Autodesk Inventor part; units mm, degrees
ref_plane "YZ Plane" through (0, 0, 0) normal (1, 0, 0) x (0, 1, 0)
ref_plane "XZ Plane" through (0, 0, 0) normal (0, 1, 0) x (-1, 0, 0)
ref_plane "XY Plane" through (0, 0, 0) normal (0, 0, 1) x (1, 0, 0)
sketch "Sketch1" plane through (0, 0, 0) normal (0, 0, 1) x (1, 0, 0)
  line L0 (0, 0) -> (30, 0)
  line L1 (30, 0) -> (30, 27)
  line L2 (30, 27) -> (0, 27)
  line L3 (0, 27) -> (0, 0)
  dimension "d0" = 30
  dimension "d1" = 27
extrude "Extrusion1" add sketch "Sketch1" along normal blind 3
sketch "Sketch2" plane through (0, 27, 0) normal (0, 1, 0) x (1, 0, 0)
  line L0 (0, 0) -> (0, -3)
  line L1 (0, 0) -> (30, 0)
  line L2 (0, -3) -> (10, -3)
  line L3 (10, -3) -> (10, 0)
  line L4 (10, 0) -> (0, 0)
  line L5 (0, 0) -> (0, -3)
  dimension "d4" = 10
extrude "Extrusion2" add sketch "Sketch2" along normal blind 2
sketch "Sketch3" plane through (0, 29, 0) normal (0, 1, 0) x (1, 0, 0)
  line L0 (0, 0) -> (0, -3)
  line L1 (0, -3) -> (32, -3)
  line L2 (32, -3) -> (32, 0)
  line L3 (32, 0) -> (0, 0)
  line L4 (0, 0) -> (0, -3)
  point P0 (30, 0)
  dimension "d7" = 2
extrude "Extrusion3" add sketch "Sketch3" along normal blind 2
chamfer "Chamfer1" distance 2 angle 45 1 edges at (0, 31, 1.5)
sketch "Sketch4" plane through (0, 0, 3) normal (0, 0, 1) x (1, 0, 0)
  line L0 (32, 29) -> (10, 29)
  line L1 (10, 29) -> (30, 24.9996)
  line L2 (10, 27) -> (10, 29)
  line L3 (30.3923, 26.9608) -> (10, 29)
  line L4 (10, 29) -> (10.3923, 30.9612) construction
  line L5 (10.3923, 30.9612) -> (30.3923, 26.9608) construction
  line L6 (30, 0) -> (30, 27)
  line L7 (30, 24.9996) -> (30.3923, 26.9608)
  point P0 (0, 0)
  dimension "d35" = 2
  dimension "d36" = 2
extrude "Extrusion4" cut sketch "Sketch4" against normal through all contours L3 L6 L1
sketch "Sketch5" plane through (0, 0, 3) normal (0, 0, 1) x (1, 0, 0)
  line L0 (2, 31) -> (32, 31)
  line L1 (26, 31) -> (28, 31)
  line L2 (28, 31) -> (28, 33)
  line L3 (28, 33) -> (26, 33)
  line L4 (26, 33) -> (26, 31)
  line L5 (30, 0) -> (30, 24.9996)
  point P0 (0, 0)
  dimension "d16" = 2
  dimension "d17" = 2
  dimension "d18" = 2
extrude "Extrusion5" add sketch "Sketch5" against normal blind 3
sketch "Sketch6" plane through (0, 0, 3) normal (0, 0, 1) x (1, 0, 0)
  line L0 (30, 0) -> (30, 24.9996)
  line L1 (30, 17.1545) -> (32, 15.9998)
  line L2 (32, 15.9998) -> (32, 8.9998)
  line L3 (32, 8.9998) -> (30, 7.8451)
  line L4 (30, 8.9998) -> (31, 9.5772)
  line L5 (31, 9.5772) -> (31, 15.4225)
  line L6 (31, 15.4225) -> (30, 15.9998)
  line L7 (30, 7.8451) -> (30, 8.9998)
  line L8 (30, 17.1545) -> (30, 15.9998)
  point P0 (0, 0)
  point P1 (32, 12.4998)
  point P2 (30, 12.4998)
  dimension "d27" = 120
  dimension "d29" = 120
  dimension "d30" = 2
  dimension "d31" = 7
  dimension "d32" = 1
extrude "Extrusion6" add sketch "Sketch6" against normal blind 3 contours L0 L4 L5 L6 L1 L2 L3
properties part number "TA11" material "ABS Plastic"
Design review of the part built by this model. Coordinates are the model's own, in mm. A direction names the side the tool comes from. Give positions to 0.01 mm unless a question says otherwise; leave off trailing zeros. Loops run counter-clockwise (first coordinate to the right, second up) from the corner with the lowest first, then second, coordinate; pieces in that order, holes last. Notation, with made-up numbers: (-32.75, 30.5) - (17.25, 30.5) arc R30 cw to (17.25, 52.5) - close; hole circle Ø10 at (39.5, 12). An arc over 180 degrees is marked (long way). Use CSV: the item, a comma, the result in double quotes. Start each with the question number.
1. Machinability: for faces 1 (the flat face through (25, 26, 2)), 2 (the flat face through (14, 31, 1)), 3 (the flat face through (30, 4, 1)), 4 (the flat face through (28, 32, 2)), which of the approach directions +Z, -Z, +X, -X, +Y, -Y give a long, thin tool a straight path to every point of the face, cutting with its end or side? Answer none if there is none.
2. Draft analysis for pull direction X (two halves, no side actions). For faces 5 (the flat face through (30, 12, 1)), 6 (the flat face through (26, 32, 2)), 7 (the flat face through (30, 31, 1)), state which applies: released by +X, released by -X, zero draft, split by the parting line, or undercut.
3. Add section C-C (y = 24). State the section outline as (x, z) points.
4. Add section A-A (x = 18). State the section outline as (y, z) points, plus the area to 3 significant figures.
5. Wall thickness on L1, parallel to X at y = 10.5, z = 0.75; L2, parallel to X at y = 3, z = 0.75; L3, parallel to Y at x = 4, z = 2.05: over which ranges is each line inside the solid? List them lowest first.
6. Insertion check: P1, Ø0.9, axis at y = 3.5, z = 2, coming from the +X side; P2, Ø1, axis at x = 25, z = 1.5, coming from the +Y side; P3, Ø2, axis at x = 24, y = 29, coming from the -Z side; P4, Ø1.6, axis at y = 28, z = 1, coming from the +X side. Each pin has a flat end and moves straight along its axis. Give the tip position at first contact, or say it passes through.
7. Add section D-D (x = 27). State the section outline as (y, z) points.
8. Add section B-B (z = 1.1). State the section outline as (x, y) points.
Results found:
1,face 1,"+Z, -Z, +X"
1,face 2,"+Z, -Z, -X, +Y"
1,face 3,"+Z, -Z, +X, -Y"
1,face 4,"+Z, -Z, +X, +Y"
2,face 5,"undercut"
2,face 6,"released by -X"
2,face 7,"zero draft"
3,outline,"(0, 0) - (30, 0) - (30, 3) - (0, 3) - close"
4,outline,"(0, 0) - (27, 0) - (27, 3) - (0, 3) - close; (29, 0) - (31, 0) - (31, 3) - (29, 3) - close"
4,area,"87.0 mm²"
5,L1,"x = 0 to 30, 31 to 32"
5,L2,"x = 0 to 30"
5,L3,"y = 0 to 31"
6,P1,"stops at x = 30"
6,P2,"stops at y = 31"
6,P3,"stops at z = 0"
6,P4,"stops at x = 10"
7,outline,"(0, 0) - (25.6, 0) - (25.6, 3) - (0, 3) - close; (29, 0) - (33, 0) - (33, 3) - (29, 3) - close"
8,outline,"(0, 0) - (30, 0) - (30, 7.85) - (32, 9) - (32, 16) - (30, 17.15) - (30, 25) - (20, 27) - (10, 27) - (10, 29) - (32, 29) - (32, 31) - (28, 31) - (28, 33) - (26, 33) - (26, 31) - (2, 31) - (0, 29) - close; hole (30, 9) - (31, 9.58) - (31, 15.42) - (30, 16) - close"
